```python
from build123d import *

# Parameters (mm, degrees)
SKETCH_1_R      = 1.9
EXTRUDE_1_DEPTH = 1.8
FILLET_1_R      = 2


with BuildPart() as part:
    # 草图1 → 凸台-拉伸1 (new body)
    with BuildSketch(Plane(origin=(0, 0, 0), x_dir=(1, 0, 0), z_dir=(0, 1, 0))):
        Polygon((0, -14), (8, -14), (8, -30), (22, -30), (22, -14), (30, -14), (30, 0), (0, 0), align=None)
        with Locations(Location((7, -7, 0), (0, 0, 270))):
            Circle(SKETCH_1_R, mode=Mode.SUBTRACT)
        with Locations(Location((23, -7, 0), (0, 0, 270))):
            Circle(SKETCH_1_R, mode=Mode.SUBTRACT)
        with Locations(Location((15, -23.124515497, 0), (0, 0, 270))):
            Circle(SKETCH_1_R, mode=Mode.SUBTRACT)
    extrude(amount=EXTRUDE_1_DEPTH)

    # 圆角1
    fillet_1_edges = [part.edges().sort_by_distance(p)[0] for p in [
        (0, 0.9, 0),
        (30, 0.9, 0),
        (30, 0.9, 14),
        (22, 0.9, 30),
        (8, 0.9, 30),
        (0, 0.9, 14),
    ]]
    fillet(fillet_1_edges, radius=FILLET_1_R)


solid = part.part
```
Here's how the part is built. I have some questions about the finished solid (model axes, mm). A direction names the side the tool comes from. Coordinates: 2 decimals unless noted, no trailing zeros. Loops run counter-clockwise (first coordinate to the right, second up) from the corner with the lowest first, then second, coordinate; pieces in that order, holes last. Notation, with made-up numbers: (-9.5, 16) - (24.5, 16) arc R23 cw to (24.5, 26) - close; hole circle Ø9 at (29.25, 88.5). An arc over 180 degrees is marked (long way). Answer as CSV lines item,"result".
Q1. If I drill on L1, parallel to X at y = 0.55, z = 7; L2, parallel to X at y = 0.6, z = 23.25; L3, parallel to X at y = 0.8, z = 15.5, over which ranges is the centre line in solid material (lowest first)? Write a range as [from, to].
Response:
L1,"[0, 5.1], [8.9, 21.1], [24.9, 30]"
L2,"[8, 13.1], [16.9, 22]"
L3,"[8, 22]"
Q2. We'd pull the mould along Z, two halves only. Please class faces 1 (the face through (22, 1, 21)), 2 (the face through (8.284, 0.887, 5.6)), 3 (the face through (29.4, 0.91, 0.57)), 4 (the face through (15, 1, 30)): pulls with the +Z half, pulls with the -Z half, needs draft (parallel to the pull), parting line crosses it, or undercut.
Response:
face 1,"needs draft"
face 2,"undercut"
face 3,"pulls with the -Z half"
face 4,"pulls with the +Z half"
Q3. For faces 5 (the face through (25, 1, 14)), 6 (the face through (8, 1, 21)), 7 (the face through (16.28, 0.89, 21.72)), which set-ups out of +Z, -Z, +X, -X, +Y, -Y let a thin tool reach every point of the face, with its end or its side?
Response:
face 5,"+Z, +X, +Y, -Y"
face 6,"+Z, -X, +Y, -Y"
face 7,"+Y, -Y"
Q4. If we section it at B-B, the plane z = 7: Write out the boundary of the cut face in (x, y), and give its area (3 significant figures).
Response:
outline,"(0, 0) - (5.1, 0) - (5.1, 1.8) - (0, 1.8) - close; (8.9, 0) - (21.1, 0) - (21.1, 1.8) - (8.9, 1.8) - close; (24.9, 0) - (30, 0) - (30, 1.8) - (24.9, 1.8) - close"
area,"40.3 mm2"
Q5. If we section it at D-D, the plane x = 15: Write out the boundary of the cut face in (y, z), and give its area (3 significant figures).
Response:
outline,"(0, 0) - (1.8, 0) - (1.8, 21.22) - (0, 21.22) - close; (0, 25.02) - (1.8, 25.02) - (1.8, 30) - (0, 30) - close"
area,"47.2 mm2"
Q6. For pin 1 (0.9 mm diameter, centred on y = 0.5, z = 22, fed in from +X); pin 2 (3.5 mm diameter, centred on x = 15, z = 23.12, fed in from -Y); pin 3 (0.5 mm diameter, centred on y = 1, z = 18.5, fed in from -X), each with a flat end and sliding along its axis, tell me the tip position at first contact or that it passes through.
Response:
pin 1,"x = 22"
pin 2,"through"
pin 3,"x = 8"
Q7. If we section it at C-C, the plane y = 0.75: Write out the boundary of the cut face in (x, z).
Response:
outline,"(0, 2) arc R2 ccw to (2, 0) - (28, 0) arc R2 ccw to (30, 2) - (30, 12) arc R2 ccw to (28, 14) - (22, 14) - (22, 28) arc R2 ccw to (20, 30) - (10, 30) arc R2 ccw to (8, 28) - (8, 14) - (2, 14) arc R2 ccw to (0, 12) - close; hole circle Ø3.8 at (7, 7); hole circle Ø3.8 at (15, 23.12); hole circle Ø3.8 at (23, 7)"
Q8. If we section it at A-A, the plane x = 23: Write out the boundary of the cut face in (y, z).
Response:
outline,"(0, 0) - (1.8, 0) - (1.8, 5.1) - (0, 5.1) - close; (0, 8.9) - (1.8, 8.9) - (1.8, 14) - (0, 14) - close"
